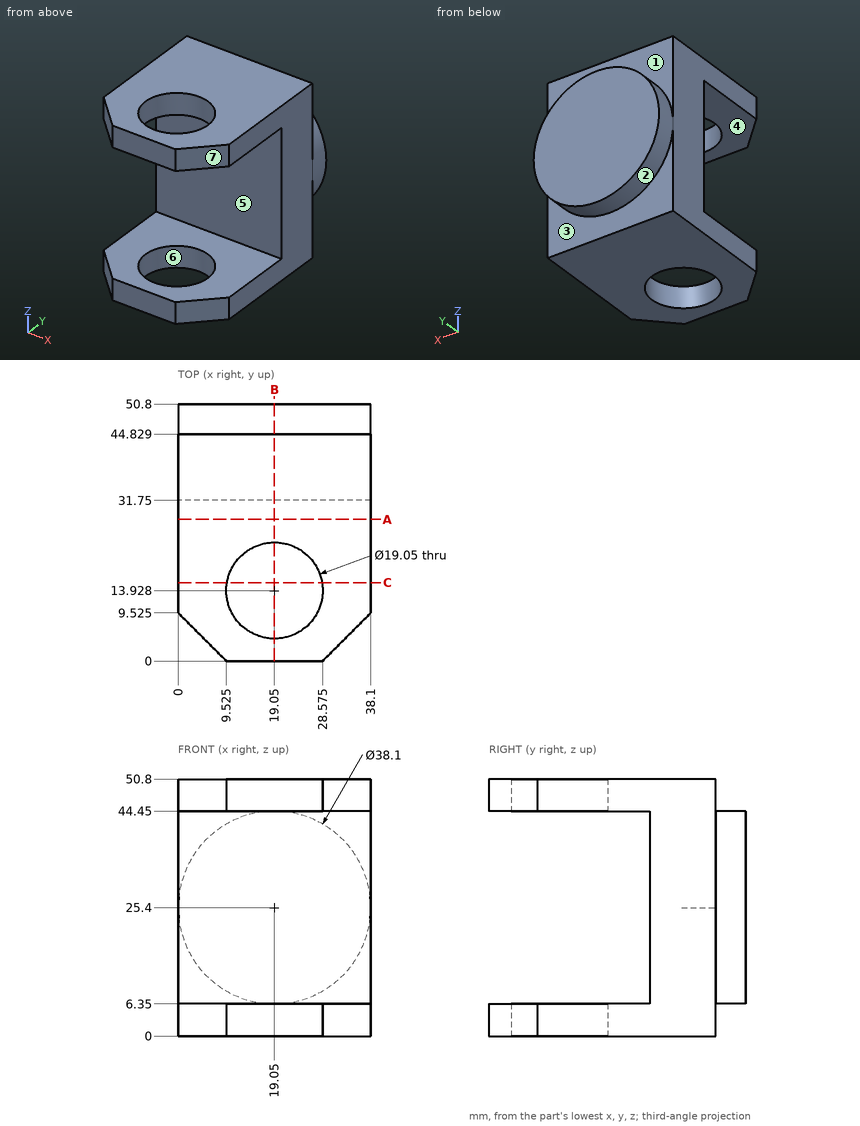
Study the drawing (mm; zero at the part's minimum x, y, z) and answer. A direction names the side the tool comes from. Give positions to 0.01 mm unless a question says otherwise; leave off trailing zeros. Write each loop counter-clockwise with the first axis right and the second up, starting at its lowest first coordinate (ties: lowest second). Pieces come first, ordered by that corner, then holes.
Item 1: Which of the six approach directions +Z, -Z, +X, -X, +Y, -Y give full straight-line access (tool end or side, diameter ignored) to the marked faces 1, 2, 3 and 4?
Item 2: Section C-C, the plane y = 15.5 is taken. Count the separate pieces of the cut face and the enclosed holes in it, plus the area to 3 significant figures.
Item 3: Flat-ended cylindrical pins translate along their axes: P1, Ø6, axis at x = 14.5, y = 20.5, coming from the +Z side; P2, Ø4, axis at x = 10, z = 33, coming from the -Y side; P3, Ø6, axis at y = 7, z = 9.5, coming from the -X side. Find the tip coordinate at first contact, or state that the pin passes through.
Item 4: Determine the mould class of the marked faces 5, 6 and 7 for opening direction X: released by +X, released by -X, zero draft, split by the parting line, or undercut.
Item 5: Find the intervals of material crossed by line 1 along Z through (x, y) = (25, 31); line 2 along Y through (x, z) = (19.05, 4.25); line 3 along Y through (x, z) = (30.5, 10), in increasing order.
Item 6: Section A-A, the plane y = 28 is taken. Write down the section's boundary in (x, z), plus the area to 3 significant figures.
Item 7: Section B-B, the plane x = 19.05 is taken. Write down the section's boundary in (y, z), plus the area to 3 significant figures.
Completed:
1. face 1: +Z, +Y
1. face 2: +Y
1. face 3: -Z, +Y
1. face 4: +X, -X, -Y
2. separate pieces: 4
2. enclosed holes: 0
2. area: 245 mm2
3. P1: stops at z = 50.8
3. P2: stops at y = 31.75
3. P3: passes through
4. face 5: zero draft
4. face 6: undercut
4. face 7: released by +X
5. line 1: z = 0 to 6.35, 44.45 to 50.8
5. line 2: y = 0 to 4.4, 23.45 to 44.83
5. line 3: y = 31.75 to 44.83
6. outline: (0, 0) - (38.1, 0) - (38.1, 6.35) - (0, 6.35) - close; (0, 44.45) - (38.1, 44.45) - (38.1, 50.8) - (0, 50.8) - close
6. area: 484 mm2
7. outline: (0, 0) - (4.4, 0) - (4.4, 6.35) - (0, 6.35) - close; (0, 44.45) - (4.4, 44.45) - (4.4, 50.8) - (0, 50.8) - close; (23.45, 0) - (44.83, 0) - (44.83, 6.35) - (50.8, 6.35) - (50.8, 44.45) - (44.83, 44.45) - (44.83, 50.8) - (23.45, 50.8) - (23.45, 44.45) - (31.75, 44.45) - (31.75, 6.35) - (23.45, 6.35) - close
7. area: 1,050 mm2
